Autodesk Inventor part; units mm, degrees
ref_plane "Work Plane1" through (1.525, 0, 0) normal (0, 0, 1) x (1, 0, 0)
ref_plane "YZ Plane" through (0, 0, 0) normal (1, 0, 0) x (0, 1, 0)
ref_plane "XZ Plane" through (0, 0, 0) normal (0, 1, 0) x (-1, 0, 0)
sketch "Sketch1" plane through (0, 0, 0) normal (0, 0, 1) x (1, 0, 0)
  line L0 (0, 5.5626) -> (0, 3.175)
  line L1 (4.2672, 3.175) -> (15.875, 3.175)
  line L2 (15.875, 3.175) -> (15.875, 0)
  line L3 (15.875, 0) -> (-0.6351, 0)
  line L4 (-3.9371, 0) -> (19.177, 0)
  line L5 (-0.6351, 0) -> (-0.6351, 5.5626)
  line L6 (-0.6351, 5.5626) -> (0, 5.5626)
  line L7 (4.2672, 3.175) -> (0.0024, 3.175)
  line L8 (0.0024, 3.175) -> (0, 3.175)
  line L9 (0, -1.1125) -> (0, 6.6751)
  dimension "d0" = 15.875
  dimension "d1" = 11.6078
  dimension "d2" = 6.35
  dimension "d9" = 0.6351
  dimension "d10" = 11.1252
  dimension "d13" = 4.2648
  dimension "d14" = 6.35
revolve "Body" add sketch "Sketch1" angle 360 about axis through (15.875, 0, 0) along (-1, 0, 0)
sketch "Sketch2" plane through (-0.6351, 0, 0) normal (-1, 0, 0) x (0, 0, 1)
  line L0 (0, 6.4231) -> (5.5626, 3.2116)
  line L1 (5.5626, 3.2116) -> (5.5626, -3.2116)
  line L2 (5.5626, -3.2116) -> (0, -6.4231)
  line L3 (0, -6.4231) -> (-5.5626, -3.2116)
  line L4 (-5.5626, -3.2116) -> (-5.5626, 3.2116)
  line L5 (-5.5626, 3.2116) -> (0, 6.4231)
  point P0 (0, 0)
  point P1 (0, 0)
  dimension "d11" = 11.1252
extrude "Head" add sketch "Sketch2" along normal blind 3.5052
sketch "Sketch4" plane through (0, 0, 0) normal (0, 0, 1) x (1, 0, 0)
  line L0 (-4.1403, 5.5626) -> (-4.1403, 6.4231)
  line L1 (-4.1403, 6.4231) -> (-3.6435, 6.4231)
  line L2 (-3.6435, 6.4231) -> (-4.1403, 5.5626)
  line L3 (-4.8413, 0) -> (0.0659, 0)
  line L4 (-0.6351, 6.4231) -> (-4.1403, 6.4231)
  line L5 (-4.1403, 3.2116) -> (-4.1403, 6.4231)
  dimension "d5" = 30
  dimension "d19" = 11.1252
revolve "Chamfer1" cut sketch "Sketch4" angle 360 about axis through (-10, 0, 0) along (1, 0, 0)
thread "Thread"
chamfer "Chamfer2" distance 0.779 distance2 0.7791 1 edges at (15.875, -3.175, 0) measured on face at (15.875, -0.7017, 0.0433)
ref_plane "Work Plane1" through (1.525, 0, 0) normal (0, 0, 1) x (1, 0, 0)
equation "\"d0\" = NLG"
equation "\"d1\" = GEL"
equation "\"d2\" = GD"
equation "\"d10\" = SD2"
equation "\"d14\" = BDM"
equation "\"d11\" = SW"
equation "\"d3\" = KOH - SD"
equation "\"d5\" = ANG1"
equation "\"d19\" = SW0"
equation "\"d15\" = GEL"
equation "\"d6\" = -0.5 * SPD + 0.5 * GD"
equation "\"NLG\" = 15.875"
equation "\"GD\" = 6.35"
equation "\"BDM\" = 6.35"
equation "\"KOH\" = 4.1402"
equation "\"GEL\" = 11.6078"
equation "\"SW\" = 11.1252"
equation "\"SW0\" = SW"
equation "\"SPD\" = GD1"
equation "\"SD2\" = SW"
equation "\"SD\" = 0.635"
equation "\"ANG1\" = 30deg"
equation "\"GAL\" = 4.26466"
equation "\"GUL\" = 0.77902"
equation "\"RR\" = 0.381"
equation "\"WFT\" = SD"
equation "\"GD1\" = 4.79196"
equation "\"THREADDIA\" = 6.35"
equation "\"SDH\" = SW"
equation "\"SDHG\" = 0.00254"
equation "\"TOA\" = 30deg"
equation "\"FAWI\" = 45deg"
equation "\"NND\" = 6.35"
equation "\"E0\" = 12.84961"
properties part number "AS 2465 - 1/4 x 5/8  UNC" material "Steel, Mild"
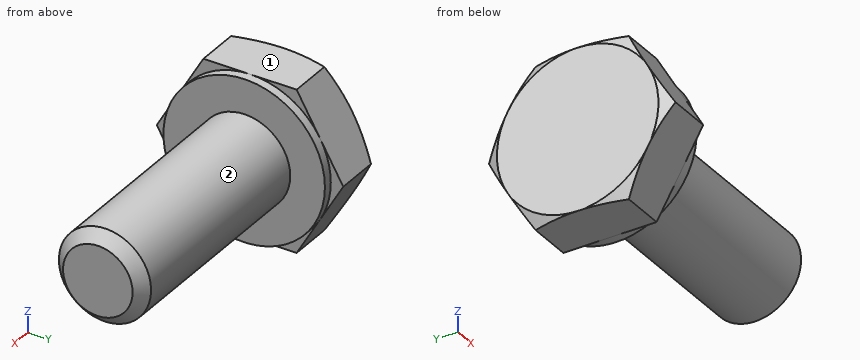
Check sheet for the modelled part. Datum: model origin and axes. Units: mm. Face numbers are marked on the shaded views. A direction names the side the tool comes from. Round coordinates to 2 decimals unless told otherwise and drop trailing zeros. Loops run counter-clockwise (first coordinate to the right, second up) from the corner with the lowest first, then second, coordinate; pieces in that order, holes last. Notation, with made-up numbers: (9, 57.25) -> (54, 57.25) arc R28 cw to (54, 96.25) -> close; hole circle Ø10 at (-0.5, -20). An arc over 180 degrees is marked (long way). Answer in a Markdown table with one row per item.
Q1. Thickness scan on L1, parallel to X at y = -3, z = 4.5; L2, parallel to Y at x = 14, z = 0 (3 decimals); L3, parallel to Y at x = -2, z = -1.5. Record the ranges inside material, lowest first.
Data:
| item | result |
|---|---|
| L1 | x = -4.14 to 0 |
| L2 | y = -3.175 to 3.175 |
| L3 | y = -5.56 to 5.56 |
Q2. Set-up check for the marked faces 1 and 2: record each of +Z, -Z, +X, -X, +Y, -Y from which the full face is reachable in a straight line by a thin tool's end or side.
Data:
| item | result |
|---|---|
| face 1 | +Z, +X, -X, +Y, -Y |
| face 2 | +X |
Q3. Go/stop test with flat-tipped pins: P1, Ø0.8, axis at y = -2.5, z = 4.5, coming from the +X side; P2, Ø3, axis at x = 9.5, z = -0.5, coming from the -Y side (3 decimals); P3, Ø2, axis at x = 6.5, z = -0.5, coming from the +Y side (3 decimals). Record where each tip stops, or that it passes through.
Data:
| item | result |
|---|---|
| P1 | stops at x = 0 |
| P2 | stops at y = -3.175 |
| P3 | stops at y = 3.175 |
Q4. Sectioned sample at A-A on x = 8.5. Enter the section's corners in (y, z) (3 decimals).
Data:
| item | result |
|---|---|
| outline | circle Ø6.35 at (0, 0) |
Q5. Sectioned sample at B-B on x = -1.75. Enter the section's corners in (y, z).
Data:
| item | result |
|---|---|
| outline | (-6.42, 0) -> (-3.21, -5.56) -> (3.21, -5.56) -> (6.42, 0) -> (3.21, 5.56) -> (-3.21, 5.56) -> close |
